from build123d import *

# Parameters (mm, degrees)
F0_W     = 57.15
F0_H     = 38.1
F1_DEPTH = 31.75
F3_DEPTH = 31.75
F5_DEPTH = 31.75


# Not quite as in the source:
# - a length typed as a fraction of an inch, garbled in the dataset ("3 / 203.2 mm" for 3/8 in), is restored
# - a feature names something its author has since deleted; it is built from what else it names


with BuildPart() as f1:
    # F0 (on Front) → F1 (new body)
    with BuildSketch(Plane.XZ):
        with Locations((28.575, 19.05)):
            Rectangle(F0_W, F0_H)
    extrude(amount=F1_DEPTH)

    # F2 (on face) → F3 (cut)
    with BuildSketch(Plane.XZ.offset(31.75)):
        with BuildLine():
            Line((57.15, 38.1), (38.1, 38.1))
            ThreePointArc((38.1, 38.1), (46.2145934678, 27.1645934678), (57.15, 19.05))
            Line((57.15, 19.05), (57.15, 38.1))
        make_face()
    extrude(amount=-F3_DEPTH, mode=Mode.SUBTRACT)

    # F4 (on face) → F5 (cut)
    with BuildSketch(Plane.XZ.offset(31.75)):
        with BuildLine():
            Line((0, 38.1), (0, 25.4))
            ThreePointArc((0, 25.4), (3.7197438789, 34.3802561211), (12.7, 38.1))
            Line((12.7, 38.1), (0, 38.1))
        make_face()
    extrude(amount=-F5_DEPTH, mode=Mode.SUBTRACT)


solid = f1.part
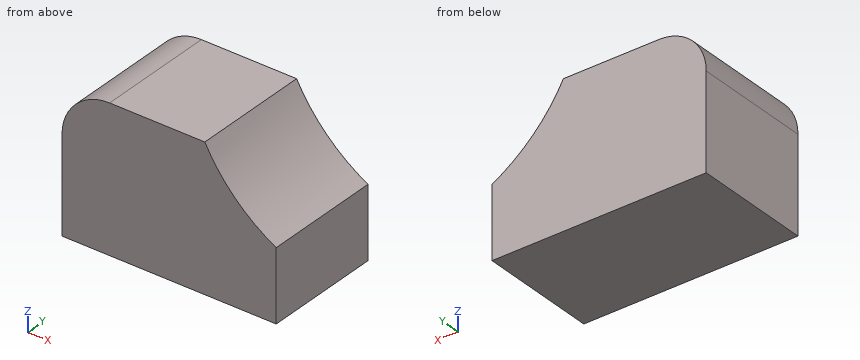
Geometry: final body of the model. Coordinates: model frame, mm. Coordinates: 2 decimals unless noted, no trailing zeros. Loops run counter-clockwise (first coordinate to the right, second up) from the corner with the lowest first, then second, coordinate; pieces in that order, holes last. Notation, with made-up numbers: (-31, 64.25) - (0, 64.25) arc R26 cw to (0, 90.25) - close; hole circle Ø3 at (-38, 52). An arc over 180 degrees is marked (long way). Put each result on its own line as item: value. Start each with the question number.
Q1. Cut plane C-C, the plane z = 20. Return loops of the section in (x, y).
Q2. Pin query (flat end, axial travel): pin 1 Ø1 at (y, z) = (-20.5, 31) entering from +X; pin 2 Ø1 at (y, z) = (-24, 21) entering from -X. Return the tip coordinate at first contact, or that it passes through.
Q3. Line query: line 1 (Z direction, x = 9, y = -16); line 2 (X direction, y = -13, z = 20); line 3 (X direction, y = -21, z = 34). Output: solid intervals per line, ascending.
Q4. Cut plane A-A, the plane y = -12.5. Return loops of the section in (x, z).
Q5. Cut plane B-B, the plane x = 8. Return loops of the section in (y, z).
Filled sheet:
1. outline: (0, -31.75) - (55.46, -31.75) - (55.46, 0) - (0, 0) - close
2. pin 1: x = 43.19
2. pin 2: x = 0
3. line 1: 0 to 37.55
3. line 2: 0 to 55.46
3. line 3: 3.35 to 40.57
4. outline: (0, 0) - (57.15, 0) - (57.15, 19.05) arc R46.48 cw to (38.1, 38.1) - (12.7, 38.1) arc R12.7 ccw to (0, 25.4) - close
5. outline: (-31.75, 0) - (0, 0) - (0, 37.2) - (-31.75, 37.2) - close
